from build123d import *

# Parameters (mm, degrees)
F1_DEPTH = 2.5
F2_SIZE  = 2


with BuildPart() as f1:
    # F0 (on Front) → F1 (new body)
    with BuildSketch(Plane.XZ):
        with BuildLine():
            Line((20, 6.4983939247), (0, 21.0292444848))
            Line((0, 21.0292444848), (-20, 6.4983939247))
            Line((-20, 6.4983939247), (-19.1806086697, 3.976566717))
            Line((-19.1806086697, 3.976566717), (-3.1309868579, 3.976566717))
            ThreePointArc((-3.1309868579, 3.976566717), (-2.5524079103, 13.3702738348), (5.5, 8.4983939247))
            ThreePointArc((5.5, 8.4983939247), (4.8718799102, 5.9459860143), (3.1309868579, 3.976566717))
            Line((3.1309868579, 3.976566717), (19.1806086697, 3.976566717))
            Line((19.1806086697, 3.976566717), (20, 6.4983939247))
        make_face()
        with BuildLine():
            Line((29.1157588363, 3.976566717), (19.1806086697, 3.976566717))
            Line((19.1806086697, 3.976566717), (17.3775660969, -1.5726277263))
            ThreePointArc((17.3775660969, -1.5726277263), (19.6325054401, -3.5904932157), (20.4695514611, -6.4983939247))
            ThreePointArc((20.4695514611, -6.4983939247), (18.5071837485, -10.6954947502), (14.02819865, -11.8809207775))
            Line((14.02819865, -11.8809207775), (12.360679775, -17.013016167))
            Line((12.360679775, -17.013016167), (-12.360679775, -17.013016167))
            Line((-12.360679775, -17.013016167), (-14.0168260009, -11.9159221924))
            ThreePointArc((-14.0168260009, -11.9159221924), (-20.236535112, -8.1998473226), (-17.388938746, -1.5376263114))
            Line((-17.388938746, -1.5376263114), (-19.1806086697, 3.976566717))
            Line((-19.1806086697, 3.976566717), (-27.784332633, 3.976566717))
            Line((-27.784332633, 3.976566717), (-27.784332633, -17.0448571444))
            Line((-27.784332633, -17.0448571444), (29.1157588363, -17.0448571444))
            Line((29.1157588363, -17.0448571444), (29.1157588363, 3.976566717))
        make_face()
        with BuildLine():
            Line((17.3775660969, -1.5726277263), (19.1806086697, 3.976566717))
            Line((19.1806086697, 3.976566717), (3.1309868579, 3.976566717))
            ThreePointArc((3.1309868579, 3.976566717), (0, 2.9983939247), (-3.1309868579, 3.976566717))
            Line((-3.1309868579, 3.976566717), (-19.1806086697, 3.976566717))
            Line((-19.1806086697, 3.976566717), (-17.388938746, -1.5376263114))
            ThreePointArc((-17.388938746, -1.5376263114), (-12.0706057057, -1.8363243506), (-9.4939811438, -6.4983939247))
            ThreePointArc((-9.4939811438, -6.4983939247), (-10.7733217403, -10.0270529523), (-14.0168260009, -11.9159221924))
            Line((-14.0168260009, -11.9159221924), (-12.360679775, -17.013016167))
            Line((-12.360679775, -17.013016167), (12.360679775, -17.013016167))
            Line((12.360679775, -17.013016167), (14.02819865, -11.8809207775))
            ThreePointArc((14.02819865, -11.8809207775), (9.7981474417, -4.8082095716), (17.3775660969, -1.5726277263))
        make_face()
    extrude(amount=F1_DEPTH)

    # F2
    f2_edges = [f1.edges().sort_by_distance(p)[0] for p in [
        (-3.130987, -2.5, 13.020221),
        (12.622434, -2.5, -11.42416),
        (-20.506019, -2.5, -6.498394),
    ]]
    chamfer(f2_edges, length=F2_SIZE)


solid = f1.part
The listing builds one solid part. Answer for the finished solid, in the listing's coordinates (mm). A direction names the side the tool comes from. Coordinates: 2 decimals unless noted, no trailing zeros. Loops run counter-clockwise (first coordinate to the right, second up) from the corner with the lowest first, then second, coordinate; pieces in that order, holes last.
1) Flat-ended cylindrical pins translate along their axes: pin 1 Ø1 at (x, y) = (-7.5, -1.5) entering from +Z; pin 2 Ø0.8 at (x, y) = (-22.5, -1) entering from +Z; pin 3 Ø12 at (x, z) = (-19, 11) entering from -Y; pin 4 Ø14.5 at (x, z) = (0, 8.5) entering from -Y. Find the tip coordinate at first contact, or state that the pin passes through.
2) Find the intervals of material crossed by L1, parallel to X at y = -1.9, z = -2; L2, parallel to Z at x = 0, y = -0.1; L3, parallel to X at y = -2.05, z = -11, in increasing order.
3) A tool of negligible diameter and unlimited length cuts with its end or side. For faces 1 (the face through (-19.596, -1.232, 5.255)), 2 (the face through (0, 0, -2)), from which of +Z, -Z, +X, -X, +Y, -Y can it reach the whole face along a straight path? Write none if from no direction.
4) Find section D-D on z = -10. Give the number of separate pieces and of enclosed holes in the cut face, then the cut area to 3 significant figures.
5) Find section B-B on y = -1.4. Write down the section's boundary in (x, z), then the cut area to 3 significant figures.
6) Find section A-A on x = 15. Write down the section's boundary in (y, z), then the cut area to 3 significant figures.
7) Determine the mould class of faces 3 (the face through (29.116, -1, -7)), 4 (the face through (0, -1, -17.045)), 5 (the face through (19.585, -1.232, 5.22)), 6 (the face through (-9.86, -1.232, 13.866)) for opening direction Z: pulls with the +Z half, pulls with the -Z half, needs draft (parallel to the pull), parting line crosses it, or undercut.
8) Find section C-C on z = 17.5. Write down the section's boundary in (x, y), then the cut area to 3 significant figures.
Values:
1. pin 1: stops at z = 15.94
1. pin 2: stops at z = 3.98
1. pin 3: stops at y = -2.5
1. pin 4: stops at y = -2.25
2. L1: x = -27.78 to -20.24, -9.76 to 9.81, 20.19 to 29.12
2. L2: z = -17.04 to 3, 14 to 21.03
2. L3: x = -27.78 to -20.43, -9.57 to 9.61, 20.39 to 29.12
3. face 1: -X, +Y, -Y
3. face 2: +Z, -Z, +X, -X, +Y
4. separate pieces: 3
4. enclosed holes: 0
4. area: 90.2 mm2
5. outline: (-27.78, -17.04) - (29.12, -17.04) - (29.12, 3.98) - (19.18, 3.98) - (20, 6.5) - (0, 21.03) - (-20, 6.5) - (-19.18, 3.98) - (-27.78, 3.98) - close; hole circle Ø12.81 at (-15, -6.5); hole circle Ø12.8 at (0, 8.5); hole circle Ø12.74 at (15, -6.5)
5. area: 1,200 mm2
6. outline: (-2.5, -17.04) - (0, -17.04) - (0, -11.97) - (-0.5, -11.97) - (-2.5, -13.97) - close; (-2.5, 0.97) - (-0.5, -1.03) - (0, -1.03) - (0, 10.13) - (-2.5, 10.13) - close
6. area: 36.6 mm2
7. face 3: needs draft
7. face 4: pulls with the -Z half
7. face 5: undercut
7. face 6: pulls with the +Z half
8. outline: (-4.86, -2.5) - (4.86, -2.5) - (4.86, 0) - (-4.86, 0) - close
8. area: 24.3 mm2
